Verification items for the finished model (mm, model axes). Round coordinates to 2 decimals unless told otherwise and drop trailing zeros. Loops run counter-clockwise (first coordinate to the right, second up) from the corner with the lowest first, then second, coordinate; pieces in that order, holes last. Notation, with made-up numbers: M -15,54 L -5,54 A26 cw -5,71 Z; hole C -3,54 d2. An arc over 180 degrees is marked long. One line per item, written item: value.
from build123d import *

# Parameters (mm, degrees)
SKETCH1_R           = 1.5
BOSS_EXTRUDE1_DEPTH = 2


with BuildPart() as part:
    # Sketch1 → Boss-Extrude1 (new body)
    with BuildSketch(Plane(origin=(0, 0, 0), x_dir=(1, 0, 0), z_dir=(0, 1, 0))):
        with BuildLine():
            Line((-16.075650118, 6.004728132), (-16.075650118, 2.004728132))
            Line((-16.075650118, 2.004728132), (23.924349882, 2.004728132))
            Line((23.924349882, 2.004728132), (23.924349882, 6.004728132))
            add(Edge.make_bspline(
                [(-16.075650118, 6.004728132), (3.924349882, 15.082742317), (23.924349882, 6.004728132)],
                knots=[0, 0, 0, 1, 1, 1], degree=2))
        make_face()
        with Locations(Location((-11.075650118, 4.004728132, 0), (0, 0, 270))):
            Circle(SKETCH1_R, mode=Mode.SUBTRACT)
        with Locations(Location((18.924349882, 4.004728132, 0), (0, 0, 90))):
            Circle(SKETCH1_R, mode=Mode.SUBTRACT)
    extrude(amount=BOSS_EXTRUDE1_DEPTH)


solid = part.part
(1) Sectioned sample at A-A on z = -4.5. Enter the section's corners in (x, y), and give its area (3 significant figures).
Completed:
outline: M -16.08,0 L -12.49,0 L -12.49,2 L -16.08,2 Z; M -9.66,0 L 17.51,0 L 17.51,2 L -9.66,2 Z; M 20.34,0 L 23.92,0 L 23.92,2 L 20.34,2 Z
area: 68.7 mm^2
(2) Mould release check, pull along Z, two halves, no side actions. Record for faces 1 (the face through (4, 1, -2.005)), 2 (the face through (-12.54, 0.99, -4.33)), 3 (the face through (17.66, 0.99, -4.81)), 4 (the face through (4, 2, -6)): +Z half, -Z half, draft (parallel to the pull), parting line (faces both ways), or undercut.
Completed:
face 1: +Z half
face 2: undercut
face 3: undercut
face 4: draft
(3) Thickness scan on L1, parallel to X at y = 0.5, z = -3.75; L2, parallel to X at y = 1.55, z = -4.5; L3, parallel to Z at x = -10, y = 1.05. Record the ranges inside material, lowest first. Write a range as from..to.
Completed:
L1: x = -16.08..-12.55, -9.6..17.45, 20.4..23.92
L2: x = -16.08..-12.49, -9.66..17.51, 20.34..23.92
L3: z = -8.34..-5.05, -2.96..-2
(4) Depth check by flat-ended pin: pin 1 Ø4 at (x, z) = (18.92, -4) entering from -Y. Enter the tip coordinate at first touch or a pass-through.
Completed:
pin 1: stops at y = 0
(5) Sectioned sample at B-B on y = 1.6. Count the separate pieces of the cut face and the enclosed holes in it, and give its area (3 significant figures).
Completed:
separate pieces: 1
enclosed holes: 2
area: 267 mm^2
